Geometry check sheet. Reference: drawing and pictorial views, mm from the part's lowest x, y, z. A direction names the side the tool comes from. Round coordinates to 2 decimals unless told otherwise and drop trailing zeros. Order: outer loops, then holes, each group sorted by start corner. A loop starts at its lowest first (then second) coordinate and runs counter-clockwise, first axis right, second up. Notation, with made-up numbers: M -37.5,3.25 L 12.5,3.25 A30 cw 12.5,25.25 Z; hole C -7.75,-27 d4. An arc over 180 degrees is marked long. Answer as a JSON object with one key per item and string values. Group by question number.
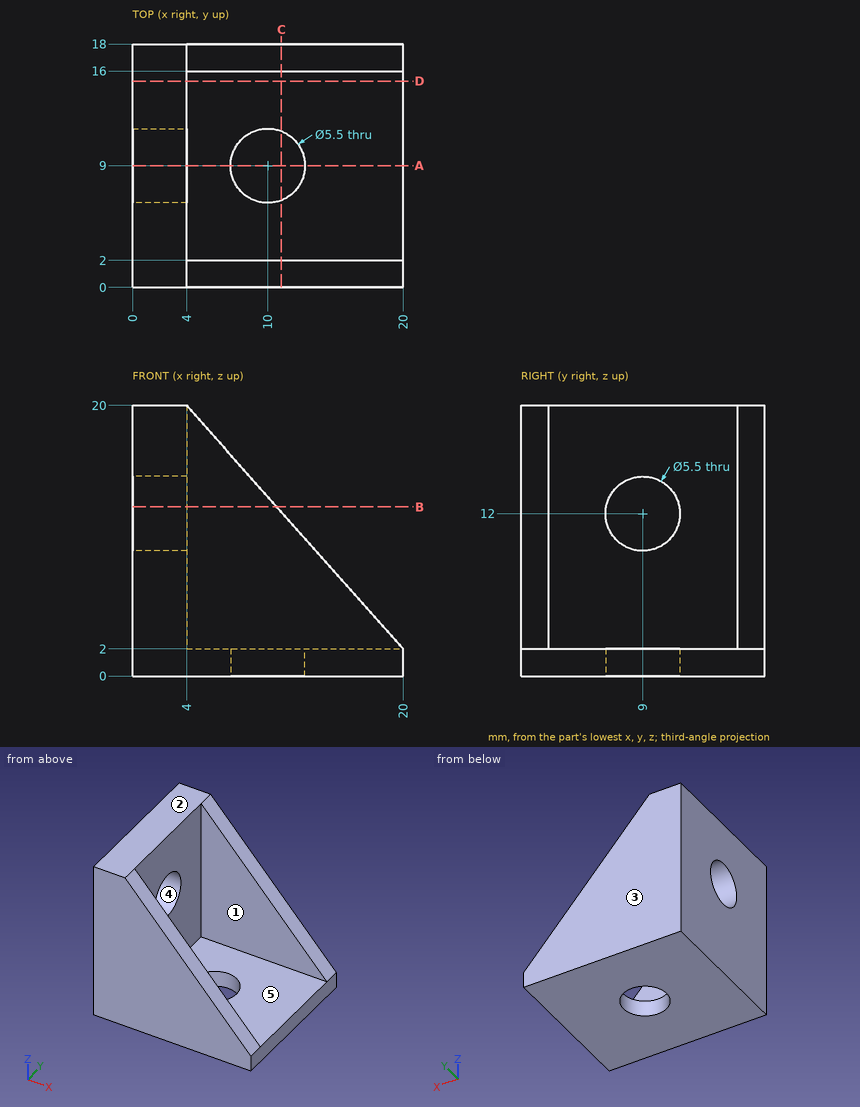
Q1. Cross-section at D-D, the plane y = 15.25. Record the cut outline in (x, z).
Q2. Tool access check on the marked faces 1 and 2. Record the directions out of +Z, -Z, +X, -X, +Y, -Y that give a thin tool (end or side, any length) a straight path to the whole face; none if there is none.
Q3. Gauge pin test, flat ends, axial feed: pin 1 Ø1.5 at (x, z) = (16.5, 9.5) entering from +Y; pin 2 Ø9 at (y, z) = (9, 12) entering from +X. Record the tip position at first contact, or that the pin passes through.
Q4. Thickness scan on line 1 (Y direction, x = 10, z = 1.4); line 2 (Z direction, x = 2.85, y = 9); line 3 (Y direction, x = 13.25, z = 4.25). Record the ranges inside material, lowest first. Write a range as from..to.
Q5. Cross-section at A-A, the plane y = 9. Record the cut outline in (x, z).
Q6. Cross-section at B-B, the plane z = 12.5. Record the cut outline in (x, y), then the cut area to 3 significant figures.
Q7. Cross-section at C-C, the plane x = 11. Record the cut outline in (y, z) (3 decimals).
Q8. Release check for a two-part mould opening along Z. For the marked faces 3, 4 and 5 record: released by +Z, released by -Z, zero draft, split by the parting line, or undercut.
Conclusion:
{
 "1": {"outline": "M 0,0 L 20,0 L 20,2 L 4,2 L 4,20 L 0,20 Z"},
 "2": {"face 1": "+Z, +X", "face 2": "+Z, +X, -X, +Y, -Y"},
 "3": {"pin 1": "through", "pin 2": "x = 4"},
 "4": {"line 1": "0..6.25, 11.75..18", "line 2": "0..9.25, 14.75..20", "line 3": "0..2, 16..18"},
 "5": {"outline": "M 0,0 L 7.25,0 L 7.25,2 L 4,2 L 4,9.25 L 0,9.25 Z; M 0,14.75 L 4,14.75 L 4,20 L 0,20 Z; M 12.75,0 L 20,0 L 20,2 L 12.75,2 Z"},
 "6": {"outline": "M 0,0 L 10.67,0 L 10.67,2 L 4,2 L 4,6.3 L 0,6.3 Z; M 0,11.7 L 4,11.7 L 4,16 L 10.67,16 L 10.67,18 L 0,18 Z", "area": "77.0 mm2"},
 "7": {"outline": "M 0,0 L 6.438,0 L 6.438,2 L 2,2 L 2,12.125 L 0,12.125 Z; M 11.562,0 L 18,0 L 18,12.125 L 16,12.125 L 16,2 L 11.562,2 Z"},
 "8": {"face 3": "zero draft", "face 4": "undercut", "face 5": "released by +Z"}
}
